Check sheet for the modelled part. Datum: model origin and axes. Units: mm. Coordinates: 2 decimals unless noted, no trailing zeros. Loops run counter-clockwise (first coordinate to the right, second up) from the corner with the lowest first, then second, coordinate; pieces in that order, holes last. Notation, with made-up numbers: (-11, 13.25) - (-7, 13.25) arc R30 cw to (-7, 37.25) - close; hole circle Ø7 at (-38.5, -11.75). An arc over 180 degrees is marked (long way). Write each question's results on one line, items separated by ' | '. Start each with the question number.
1. Cross-section at B-B (y = 2.55). Give the number of separate pieces and of enclosed holes in the cut face, and give its area (3 significant figures).
2. Thickness scan on line 1 (X direction, y = 2.55, z = 0) (3 decimals); line 2 (X direction, y = 1.75, z = 190.5); line 3 (X direction, y = 0.4, z = 59.5). Record the ranges inside material, lowest first. Write a range as [from, to].
3. Cross-section at A-A (z = 190.5). Record the cut outline in (x, y) (3 decimals).
4. Cross-section at C-C (x = 15). Record the cut outline in (y, z) (3 decimals), and give its area (3 significant figures).
5. Cross-section at D-D (z = 35.5). Record the cut outline in (x, y) (3 decimals), and give its area (3 significant figures).
Autodesk Inventor part; units mm, degrees
ref_plane "YZ Plane" through (0, 0, 0) normal (1, 0, 0) x (0, 1, 0)
ref_plane "XZ Plane" through (0, 0, 0) normal (0, 1, 0) x (-1, 0, 0)
ref_plane "XY Plane" through (0, 0, 0) normal (0, 0, 1) x (1, 0, 0)
sketch "Sketch1" plane through (0, 0, 0) normal (0, 1, 0) x (-1, 0, 0)
  line L0 (0, 0) -> (0, 190.5)
  line L1 (0, 190.5) -> (-19.3142, 47.0141)
  line L2 (-19.3142, 47.0141) -> (0, 0)
  line L3 (8.2867, -3.4607) -> (-3.4607, -8.2867)
  line L4 (-3.4607, -8.2867) -> (-25.8344, 46.1749)
  line L5 (-25.8344, 46.1749) -> (-14.0871, 51.0009)
  line L6 (-14.0871, 51.0009) -> (8.2867, -3.4607)
  line L7 (-5.4461, 197.6404) -> (7.1404, 195.9461)
  line L8 (7.1404, 195.9461) -> (-13.2479, 44.4807)
  line L9 (-13.2479, 44.4807) -> (-25.8344, 46.1749)
  line L10 (-25.8344, 46.1749) -> (-5.4461, 197.6404)
  circle A0 centre (0, 0) radius 2.5797
  circle A1 centre (-19.3142, 47.0141) radius 2.5797
  circle A2 centre (0, 190.5) radius 2.5797
  point P0 (0.8471, 196.7932)
  point P1 (2.413, -5.8737)
  point P2 (-12.7939, 47.8532)
  dimension "d0" = 150
  dimension "d1" = 190.5
  dimension "d2" = 144.78
  dimension "d3" = 12.7
  dimension "d4" = 5.1594
  dimension "d5" = 6.35
  dimension "d6" = 6.35
extrude "Extrusion1" add sketch "Sketch1" along normal blind 3.175 contours A0 L2 A1 L9 L8 L6 L0 | L0 L6 L3 L4 L9 A1 L2 A0 | L8 L6 L5 A1 L1 A2 L0 | L0 A2 L1 A1 L5 L10 L7 L8 | L8 L9 A1 L5 L6 | L9 L5 A1
fillet "Fillet1" radius 3.175 6 edges at (-7.1404, 1.5875, 195.9461) (5.4461, 1.5875, 197.6404) (25.8344, 1.5875, 46.1749) (12.7939, 1.5875, 47.8532) (3.4607, 1.5875, -8.2867) (-8.2867, 1.5875, -3.4607)
properties part number "PB OUT"
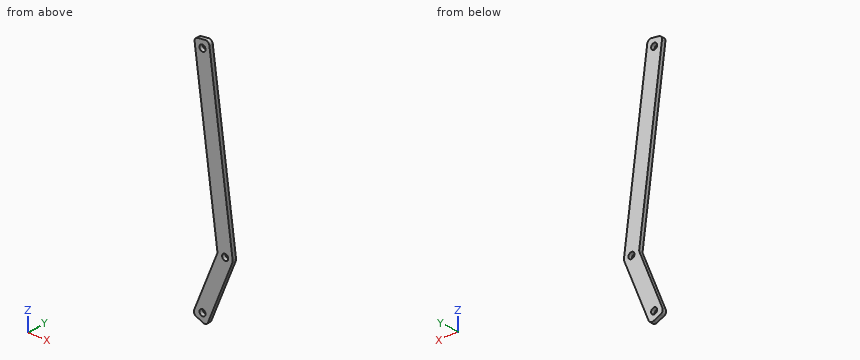
Established:
1) separate pieces: 1 | enclosed holes: 3 | area: 2,570 mm^2
2) line 1: [-6.865, -2.58], [2.58, 6.865] | line 2: [-6.41, -2.58], [2.58, 6.41] | line 3: [11.23, 24.04]
3) outline: (-6.407, 0) - (-2.58, 0) - (-2.58, 3.175) - (-6.407, 3.175) - close; (2.58, 0) - (6.407, 0) - (6.407, 3.175) - (2.58, 3.175) - close
4) outline: (0, 19.802) - (3.175, 19.802) - (3.175, 126.664) - (0, 126.664) - close | area: 339 mm^2
5) outline: (7.719, 0) - (21.449, 0) - (21.449, 3.175) - (7.719, 3.175) - close | area: 43.6 mm^2
